Autodesk Inventor part; units mm, degrees
ref_plane "YZ Plane" through (0, 0, 0) normal (1, 0, 0) x (0, 1, 0)
ref_plane "XZ Plane" through (0, 0, 0) normal (0, 1, 0) x (-1, 0, 0)
ref_plane "XY Plane" through (0, 0, 0) normal (0, 0, 1) x (1, 0, 0)
sketch "Sketch2" plane through (0, 0, 0) normal (0, 1, 0) x (-1, 0, 0)
  line L0 (0, -158.194) -> (-137, 79.097)
  line L1 (-137, 79.097) -> (137, 79.097)
  line L2 (137, 79.097) -> (0, -158.194)
  line L3 (0, -156.194) -> (-135.2679, 78.097)
  line L4 (-135.2679, 78.097) -> (135.2679, 78.097)
  line L5 (135.2679, 78.097) -> (0, -156.194)
  line L6 (0, -148.194) -> (-128.3397, 74.097)
  line L7 (-128.3397, 74.097) -> (128.3397, 74.097)
  line L8 (128.3397, 74.097) -> (0, -148.194)
  line L9 (0, 0) -> (0, -202.1847)
  line L10 (122, 72.7976) -> (-122, 72.7976)
  line L11 (-122, 72.7976) -> (-122, 81.133)
  line L12 (-122, 81.133) -> (122, 81.133)
  line L13 (122, 81.133) -> (122, 72.7976)
  line L14 (0, 72.7976) -> (0, 81.133)
  line L15 (-15, 72.7976) -> (-15, 81.133)
  line L16 (15, 72.7976) -> (15, 81.133)
  line L17 (-124.0446, 69.2563) -> (-2.0446, -142.0539)
  line L18 (-2.0446, -142.0539) -> (-9.2633, -146.2216)
  line L19 (-9.2633, -146.2216) -> (-131.2633, 65.0886)
  line L20 (-131.2633, 65.0886) -> (-124.0446, 69.2563)
  line L21 (-63.0446, -36.3988) -> (-70.2633, -40.5665)
  line L22 (-55.5446, -49.3892) -> (-62.7633, -53.5569)
  line L23 (-70.5446, -23.4084) -> (-77.7633, -27.5761)
  line L24 (2.0446, -142.0539) -> (124.0446, 69.2563)
  line L25 (124.0446, 69.2563) -> (131.2633, 65.0886)
  line L26 (131.2633, 65.0886) -> (9.2633, -146.2216)
  line L27 (9.2633, -146.2216) -> (2.0446, -142.0539)
  line L28 (63.0446, -36.3988) -> (70.2633, -40.5665)
  line L29 (70.5446, -23.4084) -> (77.7633, -27.5761)
  line L30 (55.5446, -49.3892) -> (62.7633, -53.5569)
  dimension "d34" = 1
  dimension "d35" = 5
  dimension "d36" = 274
  dimension "d37" = 0
  dimension "d51" = 15
  dimension "d52" = 15
  dimension "d53" = 15
  dimension "d54" = 30
  dimension "d57" = 360
extrude "Extrusion7" add sketch "Sketch2" along normal blind 10 contours L9 L5 L27 L2 | L0 L18 L3 L9 | L0 L22 L3 L18 | L27 L5 L30 L2 | L0 L21 L3 L22 | L30 L5 L28 L2 | L0 L23 L3 L21 | L28 L5 L29 L2 | L0 L20 L3 L23 | L29 L5 L25 L2 | L0 L1 L11 L4 L3 L20 | L25 L5 L4 L13 L1 L2 | L1 L15 L4 L11 | L13 L4 L16 L1 | L1 L14 L4 L15 | L16 L4 L14 L1
extrude "Extrusion8" add sketch "Sketch2" along normal blind 1 contours L9 L8 L27 L5 | L3 L18 L6 L9 | L3 L22 L6 L18 | L27 L8 L30 L5 | L3 L21 L6 L22 | L30 L8 L28 L5 | L3 L23 L6 L21 | L28 L8 L29 L5 | L3 L20 L6 L23 | L29 L8 L25 L5 | L3 L4 L11 L7 L6 L20 | L25 L8 L7 L13 L4 L5 | L4 L15 L7 L11 | L13 L7 L16 L4 | L4 L14 L7 L15 | L16 L7 L14 L4
fillet "Fillet3" radius 1 3 edges at (-67.634, 1, -39.0485) (67.634, 1, -39.0485) (0, 1, 78.097)
extrude "Extrusion10" cut sketch "Sketch2" along normal blind 7.5 contours L18 L19 L22 L0 | L0 L22 L3 L18 | L27 L5 L30 L2 | L2 L30 L26 L27 | L3 L22 L6 L18 | L27 L8 L30 L5 | L6 L22 L17 L18 | L27 L24 L30 L8 | L23 L19 L20 L0 | L0 L20 L3 L23 | L29 L5 L25 L2 | L2 L25 L26 L29 | L3 L20 L6 L23 | L29 L8 L25 L5 | L6 L20 L17 L23 | L29 L24 L25 L8 | L11 L12 L15 L1 | L1 L15 L4 L11 | L13 L4 L16 L1 | L1 L16 L12 L13 | L4 L15 L7 L11 | L13 L7 L16 L4 | L7 L15 L10 L11 | L13 L10 L16 L7
sketch "Sketch3" plane through (0, 0, 0) normal (0, -1, 0) x (1, 0, 0)
  line L0 (177.2057, 67.9092) -> (177.2057, 204.1642)
  line L1 (177.2057, 204.1642) -> (0, 204.1642)
  line L2 (0, 204.1642) -> (0, 67.9092)
  line L3 (61, -52.5389) -> (76, -26.5581)
  line L4 (68.5, -39.5485) -> (60.9094, -35.1661)
  line L5 (60.9094, -35.1661) -> (0, 67.9092)
  line L6 (68.5, -39.5485) -> (177.2057, 67.9092)
  point P0 (0, 0)
extrude "Extrusion11" cut sketch "Sketch3" against normal blind 1000 keep common part
sketch "Sketch4" plane through (0, 0, 74.097) normal (-1, 0, 0) x (0, 0, 1)
  line L0 (5, 0) -> (0, 0)
  line L1 (0, 0) -> (0, 7.5)
  line L2 (0, 7.5) -> (5, 7.5)
  line L3 (5, 7.5) -> (5, 0)
  point P0 (-74.097, 0)
extrude "Extrusion12" add sketch "Sketch4" against normal blind 1
sketch "Sketch5" plane through (68.5, 0, -39.5485) normal (-0.5, 0, -0.866) x (-0.866, 0, 0.5)
  line L0 (0, 0) -> (5, 0)
  line L1 (5, 0) -> (5, 7.5)
  line L2 (5, 7.5) -> (0, 7.5)
  line L3 (0, 7.5) -> (0, 0)
  point P0 (79.097, 0)
extrude "Extrusion13" add sketch "Sketch5" against normal blind 1
properties part number "Triangle"
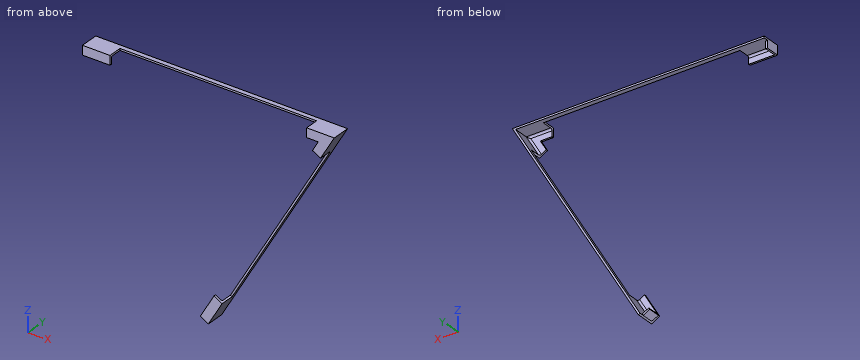
Can you work these out from the model? Positions are in its coordinate system, mm. Give positions to 0.01 mm unless a question says otherwise; leave off trailing zeros. Order: outer loops, then holes, each group sorted by start corner. A loop starts at its lowest first (then second) coordinate and runs counter-clockwise, first axis right, second up. Notation, with made-up numbers: M -17.75,82 L 30.25,82 A16 cw 30.25,92 Z; hole C 46.25,4.5 d8. An arc over 180 degrees is marked long. Use one line per item in the form item = value. Start each with the question number.
Item 1: If we section it at B-B (y = 4): Write out the boundary of the cut face in (x, z).
Item 2: Will these pins go through, and if not, where does the flat tip stop? pin 1 Ø0.5 at (x, z) = (58, 79) entering from -Y; pin 2 Ø0.8 at (x, y) = (125, 0.5) entering from -Z; pin 3 Ø12 at (x, z) = (100, -2) entering from +Y; pin 4 Ø2.5 at (x, y) = (71.5, 4) entering from -Z.
Item 3: If we section it at A-A (x = 89): Write out the boundary of the cut face in (y, z).
Item 4: If I drill on line 1 along Z through (x, y) = (9, 2); line 2 along Z through (x, y) = (84.5, 9.75); line 3 along Z through (x, y) = (71.5, 1.75), over which ranges is the centre line in solid material (lowest first)?
Item 5: If we section it at C-C (x = 30.5): Write out the boundary of the cut face in (y, z).
Item 6: If we section it at D-D (z = 1): Write out the boundary of the cut face in (x, y).
Outcome:
q1.outline = M 0,74.1 L 1,74.1 L 1,78.1 L 15,78.1 L 15,79.1 L 0,79.1 Z; M 64.17,-37.05 L 67.63,-39.05 L 68.5,-39.55 L 76,-26.56 L 75.13,-26.06 L 68.13,-38.18 L 64.67,-36.18 Z; M 122,78.1 L 135.27,78.1 L 128.63,66.61 L 129.5,66.11 L 137,79.1 L 122,79.1 Z
q2.pin_1 = 7.5
q2.pin_2 = 68.47
q2.pin_3 = through
q2.pin_4 = -36.52
q3.outline = M 7.5,-4.04 L 10,-4.04 L 10,-2.04 L 7.5,-2.04 Z; M 7.5,78.1 L 10,78.1 L 10,79.1 L 7.5,79.1 Z
q4.line_1 = 78.1 to 79.1
q4.line_2 = -11.84 to -9.84, 78.1 to 79.1
q4.line_3 = -34.35 to -32.29
q5.outline = M 7.5,78.1 L 10,78.1 L 10,79.1 L 7.5,79.1 Z
q6.outline = M 90.76,7.5 L 91.91,7.5 L 91.91,10 L 90.76,10 Z
